Could you check a few things on this model? Use its own coordinates, in mm. A direction names the side the tool comes from. Round coordinates to 2 decimals unless told otherwise and drop trailing zeros. Order: outer loops, then holes, each group sorted by start corner. A loop starts at its lowest first (then second) coordinate and runs counter-clockwise, first axis right, second up. Notation, with made-up numbers: (16, 79.25) -> (63, 79.25) arc R11 cw to (63, 93.25) -> close; hole circle Ø1 at (68.25, 71). An arc over 180 degrees is marked (long way). One line per question, with ' | ' between items.
```python
from build123d import *

# Parameters (mm, degrees)
SKETCH_1_W          = 20
SKETCH_1_H          = 20
SKETCH_1_W_2        = 18
SKETCH_1_H_2        = 18
EXTRUDE_1_DEPTH     = 250
SKETCH_2_R          = 1.65
CUT_EXTRUDE_1_DEPTH = 251.99800796


with BuildPart() as part:
    # 草图1 → 凸台-拉伸1 (new body)
    with BuildSketch(Plane.XY):
        Rectangle(SKETCH_1_W, SKETCH_1_H)
        Rectangle(SKETCH_1_W_2, SKETCH_1_H_2, mode=Mode.SUBTRACT)
    extrude(amount=EXTRUDE_1_DEPTH)

    # 草图2 → 切除-拉伸1 (cut, through all)
    with BuildSketch(Plane(origin=(0, 10, 0), x_dir=(1, 0, 0), z_dir=(0, 1, 0))):
        with Locations(Location((0, -10, 0), (0, 0, 270))):
            Circle(SKETCH_2_R)
        with Locations(Location((0, -20, 0), (0, 0, 270))):
            Circle(SKETCH_2_R)
        with Locations(Location((0, -30, 0), (0, 0, 270))):
            Circle(SKETCH_2_R)
        with Locations(Location((0, -240, 0), (0, 0, 270))):
            Circle(SKETCH_2_R)
        with Locations(Location((0, -230, 0), (0, 0, 270))):
            Circle(SKETCH_2_R)
    extrude(amount=-CUT_EXTRUDE_1_DEPTH, mode=Mode.SUBTRACT)


solid = part.part
```
1. I want a section at C-C on z = 72. List the corners of the cut face in (x, y) for me, and give its area (3 significant figures).
From the geometry:
outline: (-10, -10) -> (10, -10) -> (10, 10) -> (-10, 10) -> close; hole (-9, -9) -> (9, -9) -> (9, 9) -> (-9, 9) -> close | area: 76.0 mm²
2. If we mould it in two halves opening along Y, with no side actions, what happens to faces 1 (the face through (10, 0, 123)), 2 (the face through (0, 10, 123)), 3 (the face through (0, -9, 123))? For each: pulls with the +Y half, pulls with the -Y half, needs draft (parallel to the pull), parting line crosses it, or undercut.
From the geometry:
face 1: needs draft | face 2: pulls with the +Y half | face 3: undercut
3. I need wall thicknesses on probe 1 along X at (y, z) = (7, 238); probe 2 along X at (y, z) = (-9.4, 240). Which ranges of each line are inside material? Lowest first, please.
From the geometry:
probe 1: x = -10 to -9, 9 to 10 | probe 2: x = -10 to -1.65, 1.65 to 10
4. I want a section at A-A on y = 0.5. List the corners of the cut face in (x, z) for me, and give its area (3 significant figures).
From the geometry:
outline: (-10, 0) -> (-9, 0) -> (-9, 250) -> (-10, 250) -> close; (9, 0) -> (10, 0) -> (10, 250) -> (9, 250) -> close | area: 500 mm²
5. I'm going to push a flat-ended pin straight in: pin 1 (2 mm diameter, centred on x = 0, z = 230, fed in from -Y). Where does the tip first touch, or does it pass through?
From the geometry:
pin 1: passes through
6. On a 3-axis mill with a long thin cutter (end or side, diameter ignored), from which of +Z, -Z, +X, -X, +Y, -Y can I reach the whole of each face in a straight line? I mean faces 4 (the face through (-10, 0, 123)), 5 (the face through (0, 9, 123)). Say none if no direction works.
From the geometry:
face 4: +Z, -Z, -X, +Y, -Y | face 5: +Z, -Z
